```python
from build123d import *

# Parameters (mm, degrees)
EXTRUDE_THIN1_DEPTH            = 25
BOSS_EXTRUDE1_DEPTH            = 25
BOSS_EXTRUDE2_DEPTH            = 4
FILLET1_R                      = 10
CBORE_FOR_M4_SHCS1_D           = 4.3
CBORE_FOR_M4_SHCS1_CBORE_D     = 8
CBORE_FOR_M4_SHCS1_CBORE_DEPTH = 4
FILLET2_R                      = 5


with BuildPart() as part:
    # Sketch2 → Extrude-Thin1 (new body)
    with BuildSketch(Plane.XY):
        Polygon((239.726649941, 213.650926496), (239.696415712, 306.224679496), (390.940168333, 284.538204309), (390.956204861, 235.436188292), align=None)
        Polygon((244.724765221, 219.422538988), (244.698299899, 300.456332965), (385.941583666, 280.203800773), (385.954790061, 239.767325867), align=None, mode=Mode.SUBTRACT)
    extrude(amount=EXTRUDE_THIN1_DEPTH)

    # Sketch3 → Boss-Extrude1 (add)
    with BuildSketch(Plane.XY):
        Polygon((244.698299899, 300.456332965), (256.034798835, 298.830819854), (244.702040223, 289.003888378), align=None)
        Polygon((244.721024897, 230.874983576), (244.724765221, 219.422538988), (256.060199967, 221.055456665), align=None)
    extrude(amount=BOSS_EXTRUDE1_DEPTH)

    # Sketch4 → Boss-Extrude2 (add)
    with BuildSketch(Plane.XY.offset(25)):
        Polygon((239.696415712, 306.224679496), (390.940168333, 284.538204309), (390.956204861, 235.436188292), (239.726649941, 213.650926496), align=None)
    extrude(amount=BOSS_EXTRUDE2_DEPTH)

    # Fillet1
    fillet1_edges = [part.edges().sort_by_distance(p)[0] for p in [
        (239.726649941, 213.650926496, 14.5),
        (390.956204861, 235.436188292, 14.5),
        (390.940168333, 284.538204309, 14.5),
        (239.696415712, 306.224679496, 14.5),
    ]]
    fillet(fillet1_edges, radius=FILLET1_R)

    # CBORE for M4 SHCS1 (through all)
    with Locations(Plane(origin=(247.290055606, 297.458116912, 29), x_dir=(1, 0, 0), z_dir=(0, 0, 1))):
        with Locations((0, 0), (0.024506359, -75.035669596)):
            CounterBoreHole(CBORE_FOR_M4_SHCS1_D / 2, CBORE_FOR_M4_SHCS1_CBORE_D / 2, CBORE_FOR_M4_SHCS1_CBORE_DEPTH)

    # Fillet2
    fillet2_edges = [part.edges().sort_by_distance(p)[0] for p in [
        (385.954790061, 239.767325867, 12.5),
        (385.941583666, 280.203800773, 12.5),
        (256.034798835, 298.830819854, 12.5),
        (244.702040223, 289.003888378, 12.5),
        (244.721024897, 230.874983576, 12.5),
        (256.060199967, 221.055456665, 12.5),
    ]]
    fillet(fillet2_edges, radius=FILLET2_R)


solid = part.part
```
Read the model definition and answer for the solid it produces. Units are mm, in the model's axes. A direction names the side the tool comes from. Coordinates: 2 decimals unless noted, no trailing zeros. Order: outer loops, then holes, each group sorted by start corner. A loop starts at its lowest first (then second) coordinate and runs counter-clockwise, first axis right, second up. Notation, with made-up numbers: (30.25, 31.5) - (64.25, 31.5) arc R20 ccw to (64.25, 61.5) - close; hole circle Ø4 at (-23.5, -15). An arc over 180 degrees is marked (long way). Answer as a JSON object with one key per item and string values. Group by question number.
Item 1: Consider probe 1 along X at (y, z) = (266, 10.25); probe 2 along Z at (x, y) = (265, 267). Determine where each line is inside the solid, lowest interval first. Write a range as from..to.
Item 2: Section C-C (y = 254) is taken. Give the vertices of the cut face in (x, z).
Item 3: The mould has two halves that part along X. Classify faces 4 (the face through (250.424, 293.965, 12.325)), 5 (the face through (316, 261, 29)), 6 (the face through (388.45, 237.48, 14.3)): +X half, -X half, draft (parallel to the pull), parting line (faces both ways), or undercut.
Item 4: Flat-ended cylindrical pins translate along their axes: P1, Ø4, axis at y = 256.5, z = 6, coming from the -X side; P2, Ø8, axis at x = 299, z = 18, coming from the +Y side; P3, Ø10, axis at x = 375, z = 21.5, coming from the +Y side. Find the tip coordinate at first contact, or state that the pin passes through.
Item 5: Section B-B (x = 278.5) is taken. Give the vertices of the cut face in (y, z).
Item 6: A tool of negligible diameter and unlimited length cuts with its end or side. For faces 1 (the face through (247.781, 220.324, 12.325)), 2 (the face through (301, 260, 25)), 3 (the face through (249, 295.7, 25)), from which of +Z, -Z, +X, -X, +Y, -Y can it reach the whole face along a straight path? Write none if from no direction.
Item 7: Section A-A (z = 10.75) is taken. Give the vertices of the cut face in (x, y).
Results are:
{
 "1": {"probe 1": "x = 239.71..244.71, 385.95..390.95", "probe 2": "z = 25..29"},
 "2": {"outline": "(239.71, 0) - (244.71, 0) - (244.71, 25) - (385.95, 25) - (385.95, 0) - (390.95, 0) - (390.95, 29) - (239.71, 29) - close"},
 "3": {"face 4": "undercut", "face 5": "draft", "face 6": "+X half"},
 "4": {"P1": "stops at x = 239.71", "P2": "stops at y = 298.29", "P3": "stops at y = 287.54"},
 "5": {"outline": "(219.24, 0) - (224.29, 0) - (224.29, 25) - (295.61, 25) - (295.61, 0) - (300.66, 0) - (300.66, 29) - (219.24, 29) - close"},
 "6": {"face 1": "+Z, -Z", "face 2": "-Z", "face 3": "+Z"},
 "7": {"outline": "(239.7, 294.68) - (239.72, 225.19) arc R10 ccw to (251.15, 215.3) - (382.38, 234.2) arc R10 ccw to (390.95, 244.1) - (390.94, 275.87) arc R10 ccw to (382.36, 285.77) - (251.12, 304.59) arc R10 ccw to start; hole (244.7, 286.72) - (244.72, 233.16) arc R5 ccw to (246.45, 229.38) - (254.33, 222.55) arc R5 ccw to (258.32, 221.38) - (381.67, 239.15) arc R5 ccw to (385.95, 244.1) - (385.94, 275.87) arc R5 ccw to (381.65, 280.82) - (258.3, 298.51) arc R5 ccw to (254.31, 297.33) - (246.43, 290.5) arc R5 ccw to start; hole circle Ø4.3 at (247.29, 297.46); hole circle Ø4.3 at (247.31, 222.42)"}
}
